```python
from build123d import *

# Parameters (mm, degrees)
SKETCH1_3_R         = 1.5
SKETCH1_3_R_2       = 4
SKETCH1_3_R_3       = 2
BOSS_EXTRUDE2_DEPTH = 1.25
FILLET2_R           = 10


with BuildPart() as part:
    # Sketch1_3 → Boss-Extrude2 (new, symmetric)
    with BuildSketch(Plane.XY):
        Polygon((53.5, 37.5), (-53.5, 37.5), (-53.5, -12.5), (-25, -37.5), (25, -37.5), (53.5, -12.5), align=None)
        with Locations((0, -29.5)):
            Circle(SKETCH1_3_R, mode=Mode.SUBTRACT)
        with Locations((-16.5, -27.75)):
            Circle(SKETCH1_3_R, mode=Mode.SUBTRACT)
        with Locations((16.5, -27.75)):
            Circle(SKETCH1_3_R, mode=Mode.SUBTRACT)
        with Locations((-38.5, 17.5)):
            Circle(SKETCH1_3_R_2, mode=Mode.SUBTRACT)
        with Locations((38.5, 17.5)):
            Circle(SKETCH1_3_R_2, mode=Mode.SUBTRACT)
        with Locations((-16.5, -2.75)):
            Circle(SKETCH1_3_R_3, mode=Mode.SUBTRACT)
        with Locations((16.5, -2.75)):
            Circle(SKETCH1_3_R_3, mode=Mode.SUBTRACT)
    extrude(amount=BOSS_EXTRUDE2_DEPTH, both=True)

    # Fillet2
    fillet2_edges = [part.edges().sort_by_distance(p)[0] for p in [
        (53.5, -12.5, 0),
        (25, -37.5, 0),
        (-25, -37.5, 0),
        (-53.5, -12.5, 0),
        (-53.5, 37.5, 0),
        (53.5, 37.5, 0),
    ]]
    fillet(fillet2_edges, radius=FILLET2_R)


solid = part.part
```
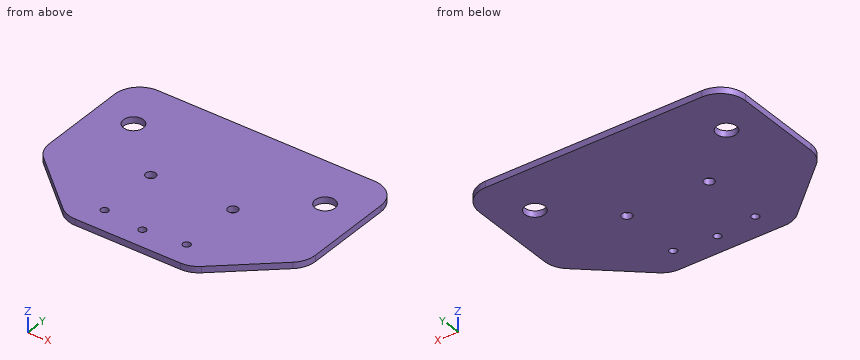
For this review, take the finished solid that the model builds, in its own axes (mm). Round coordinates to 2 decimals unless told otherwise and drop trailing zeros. Write each loop counter-clockwise with the first axis right and the second up, starting at its lowest first coordinate (ties: lowest second). Pieces come first, ordered by that corner, then holes. Notation, with made-up numbers: (-34.5, -20) -> (-11.5, -20) arc R18 ccw to (-11.5, 15) -> close; hole circle Ø1 at (23, 85.5). An arc over 180 degrees is marked (long way). One line per question, with ' | ' between items. Start each with the question number.
(1) Add section B-B, the plane x = -16.5. Write out the cut boundary in (y, z).
(2) Insertion check: P1, Ø1.5, axis at x = -24.5, z = -0.5, coming from the -Y side; P2, Ø6.5, axis at x = -16.5, y = -2.75, coming from the -Z side. Each pin has a flat end and moves straight along its axis. Give the tip position at first contact, or say it passes through.
(3) Add section A-A, the plane z = -0.7. Write out the cut boundary in (x, y).
(4) Add section D-D, the plane x = 38.5. Write out the cut boundary in (y, z).
(5) For line 1 along Y through (x, z) = (16.5, 0.1); line 2 along Y through (x, z) = (0, 0.55); line 3 along Y through (x, z) = (1, -0.7), list the stretches that pass through material, from the lowest coordinate up. Write a range as from..to.
(6) Add section C-C, the plane x = 0. Write out the cut boundary in (y, z).
Answer list:
1) outline: (-37.5, -1.25) -> (-29.25, -1.25) -> (-29.25, 1.25) -> (-37.5, 1.25) -> close; (-26.25, -1.25) -> (-4.75, -1.25) -> (-4.75, 1.25) -> (-26.25, 1.25) -> close; (-0.75, -1.25) -> (37.5, -1.25) -> (37.5, 1.25) -> (-0.75, 1.25) -> close
2) P1: y = -37.18 | P2: z = -1.25
3) outline: (-53.5, -7.97) arc R10 ccw to (-50.09, -15.49) -> (-27.83, -35.02) arc R10 ccw to (-21.24, -37.5) -> (21.24, -37.5) arc R10 ccw to (27.83, -35.02) -> (50.09, -15.49) arc R10 ccw to (53.5, -7.97) -> (53.5, 27.5) arc R10 ccw to (43.5, 37.5) -> (-43.5, 37.5) arc R10 ccw to (-53.5, 27.5) -> close; hole circle Ø8 at (-38.5, 17.5); hole circle Ø4 at (-16.5, -2.75); hole circle Ø3 at (-16.5, -27.75); hole circle Ø3 at (0, -29.5); hole circle Ø4 at (16.5, -2.75); hole circle Ø3 at (16.5, -27.75); hole circle Ø8 at (38.5, 17.5)
4) outline: (-25.66, -1.25) -> (13.5, -1.25) -> (13.5, 1.25) -> (-25.66, 1.25) -> close; (21.5, -1.25) -> (37.5, -1.25) -> (37.5, 1.25) -> (21.5, 1.25) -> close
5) line 1: -37.5..-29.25, -26.25..-4.75, -0.75..37.5 | line 2: -37.5..-31, -28..37.5 | line 3: -37.5..-30.62, -28.38..37.5
6) outline: (-37.5, -1.25) -> (-31, -1.25) -> (-31, 1.25) -> (-37.5, 1.25) -> close; (-28, -1.25) -> (37.5, -1.25) -> (37.5, 1.25) -> (-28, 1.25) -> close
